Verification items for the finished model (mm, model axes). A direction names the side the tool comes from. Round coordinates to 2 decimals unless told otherwise and drop trailing zeros. Write each loop counter-clockwise with the first axis right and the second up, starting at its lowest first coordinate (ties: lowest second). Pieces come first, ordered by that corner, then holes.
from build123d import *

# Parameters (mm, degrees)
SKETCH1_R           = 9.525
SKETCH1_W           = 3
SKETCH1_H           = 4
BOSS_EXTRUDE1_DEPTH = 2.5
SKETCH2_R           = 0.5
SKETCH2_W           = 2.1
SKETCH2_H           = 7.525
CUT_EXTRUDE1_DEPTH  = 14.700410578


with BuildPart() as part:
    # Sketch1 → Boss-Extrude1 (new body)
    with BuildSketch(Plane.XY):
        Circle(SKETCH1_R)
        Rectangle(SKETCH1_W, SKETCH1_H, mode=Mode.SUBTRACT)
    extrude(amount=BOSS_EXTRUDE1_DEPTH)

    # Sketch2 → Cut-Extrude1 (cut, through all)
    with BuildSketch(Plane.XY.offset(2.5)):
        with Locations((-1.5, -2)):
            Circle(SKETCH2_R)
        with Locations((1.5, -2)):
            Circle(SKETCH2_R)
        with Locations((0, 5.7625)):
            Rectangle(SKETCH2_W, SKETCH2_H)
    extrude(amount=-CUT_EXTRUDE1_DEPTH, mode=Mode.SUBTRACT)


solid = part.part
Q1. Sectioned sample at D-D (y = 7.25). Enter the section's corners in (x, z), plus the area to 3 significant figures.
Recorded:
outline: (-6.18, 0) - (-1.05, 0) - (-1.05, 2.5) - (-6.18, 2.5) - close; (1.05, 0) - (6.18, 0) - (6.18, 2.5) - (1.05, 2.5) - close
area: 25.6 mm2
Q2. Sectioned sample at C-C (x = 0). Enter the section's corners in (y, z) (3 decimals).
Recorded:
outline: (-9.525, 0) - (-2, 0) - (-2, 2.5) - (-9.525, 2.5) - close
Q3. Sectioned sample at B-B (z = 0.55). Enter the section's corners in (x, y) (3 decimals), plus the area to 3 significant figures.
Recorded:
outline: (-1.5, -1.5) - (-1.5, 2) - (-1.05, 2) - (-1.05, 9.467) arc R9.525 ccw (long way) to (1.05, 9.467) - (1.05, 2) - (1.5, 2) - (1.5, -1.5) arc R0.5 cw (long way) to (1, -2) - (-1, -2) arc R0.5 cw (long way) to start
area: 256 mm2
Q4. Depth check by flat-ended pin: P1, Ø1, axis at y = 1, z = 1.5, coming from the -X side; P2, Ø0.8, axis at y = 7, z = 1, coming from the -X side; P3, Ø1.5, axis at y = -6.5, z = 0.5, coming from the +X side. Enter the tip coordinate at first touch or a pass-through.
Recorded:
P1: stops at x = -9.51
P2: stops at x = -6.87
P3: stops at x = 7.59
Q5. Material ranges on line 1 along X through (y, z) = (3.25, 2.4); line 2 along X through (y, z) = (1.5, 1.65); line 3 along Y through (x, z) = (4, 1.4), recorded low to high.
Recorded:
line 1: x = -8.95 to -1.05, 1.05 to 8.95
line 2: x = -9.41 to -1.5, 1.5 to 9.41
line 3: y = -8.64 to 8.64
Q6. Tool access check on faces 1 (the flat face through (2, 0, 0)), 2 (the flat face through (-1.05, 6, 1)), 3 (the flat face through (-1.5, 0, 1)). Record the directions out of +Z, -Z, +X, -X, +Y, -Y that give a thin tool (end or side, any length) a straight path to the whole face; none if there is none.
Recorded:
face 1: -Z, +X, -X, +Y, -Y
face 2: +Z, -Z, +Y
face 3: +Z, -Z
Q7. Release check for a two-part mould opening along X. For faces 4 (the flat face through (1.5, 0, 1)), 5 (the flat face through (2, 0, 2.5)), 6 (the cylindrical face through (-0.404, -9.516, 1.232)) record: released by +X, released by -X, zero draft, split by the parting line, or undercut.
Recorded:
face 4: undercut
face 5: zero draft
face 6: split by the parting line
Q8. Sectioned sample at A-A (y = 0.75). Enter the section's corners in (x, z), plus the area to 3 significant figures.
Recorded:
outline: (-9.5, 0) - (-1.5, 0) - (-1.5, 2.5) - (-9.5, 2.5) - close; (1.5, 0) - (9.5, 0) - (9.5, 2.5) - (1.5, 2.5) - close
area: 40.0 mm2
